Part print with two shaded views. Sizes in mm from the minimum x, y, z corner. A direction names the side the tool comes from. Round coordinates to 2 decimals unless told otherwise and drop trailing zeros. Loops run counter-clockwise (first coordinate to the right, second up) from the corner with the lowest first, then second, coordinate; pieces in that order, holes last. Notation, with made-up numbers: M -28,-9.75 L -18,-9.75 A38 cw -18,29.25 Z; hole C 65.25,23.5 d7. An arc over 180 degrees is marked long. Use a Markdown table: item, result. Add a question column.
Item 1: Saw through at D-D on z = 24.13. Write the cut outline in (x, y) (1 decimal).
Item 2: Saw through at C-C on z = 36.5. Write the cut outline in (x, y) (1 decimal).
Item 3: Saw through at A-A on z = 30.48. Write the cut outline in (x, y) (1 decimal).
Item 4: Pin check, flat tips, straight feed: P1, Ø8, axis at x = 36.5, z = 34.5, coming from the -Y side; P2, Ø3.5, axis at x = 52, y = 37.5, coming from the -Z side; P3, Ø12.5, axis at y = 11, z = 20, coming from the -X side; P4, Ø11.5, axis at x = 17.5, z = 34, coming from the -Y side. Stop position of each tip, or through.
Item 5: Wall check: L1, parallel to Y at x = 40, z = 24 (1 decimal); L2, parallel to Y at x = 52.35, z = 43.18 (1 decimal); L3, parallel to X at y = 34, z = 46 (1 decimal). Give the ranges that are in metal, low to high. Write a range as from..to.
Item 6: Tool access for the marked faces 1, 2, 3 and 4: list every direction of +Z, -Z, +X, -X, +Y, -Y with a clear straight run to the whole face (end or side of a thin tool).
Item 7: Saw through at B-B on y = 12.7. Write the cut outline in (x, z) (1 decimal).
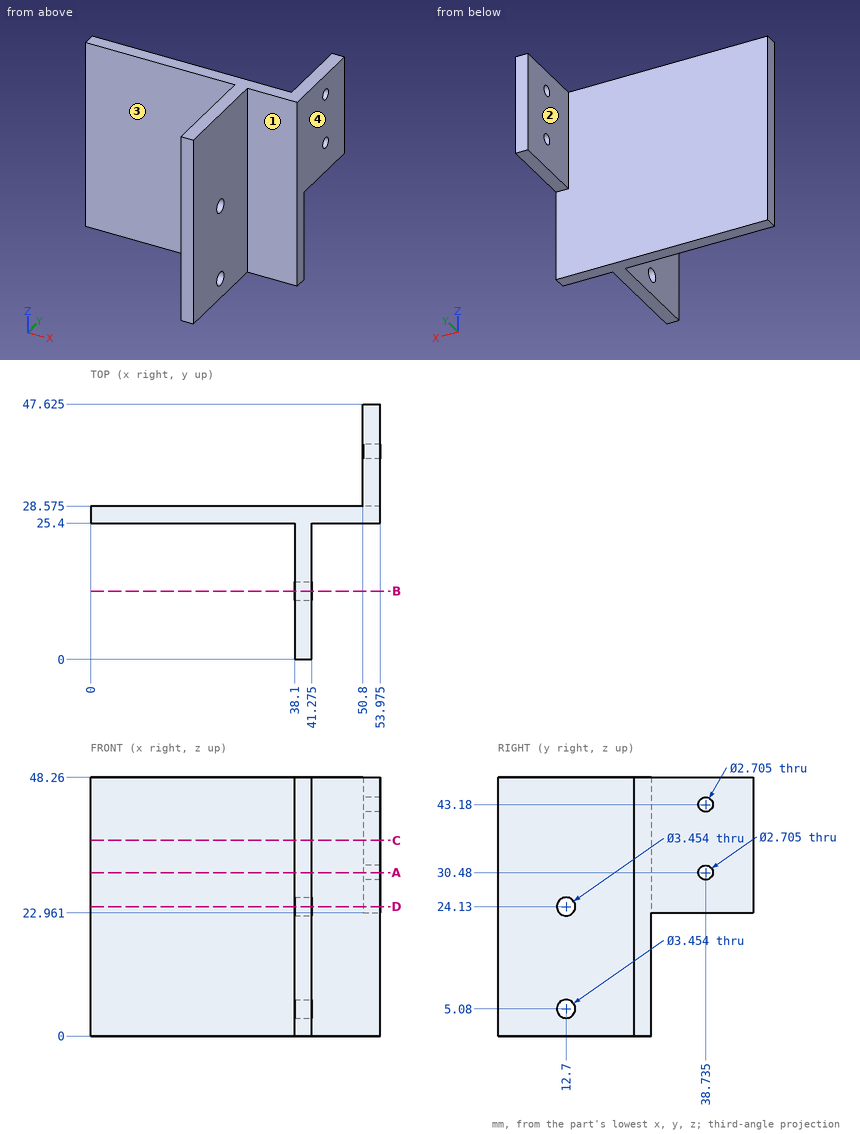
Entries:
| question | item | result |
|---|---|---|
| 1 | outline | M 0,25.4 L 38.1,25.4 L 38.1,14.4 L 41.3,14.4 L 41.3,25.4 L 54,25.4 L 54,47.6 L 50.8,47.6 L 50.8,28.6 L 0,28.6 Z; M 38.1,0 L 41.3,0 L 41.3,11 L 38.1,11 Z |
| 2 | outline | M 0,25.4 L 38.1,25.4 L 38.1,0 L 41.3,0 L 41.3,25.4 L 54,25.4 L 54,47.6 L 50.8,47.6 L 50.8,28.6 L 0,28.6 Z |
| 3 | outline | M 0,25.4 L 38.1,25.4 L 38.1,0 L 41.3,0 L 41.3,25.4 L 54,25.4 L 54,37.4 L 50.8,37.4 L 50.8,28.6 L 0,28.6 Z; M 50.8,40.1 L 54,40.1 L 54,47.6 L 50.8,47.6 Z |
| 4 | P1 | y = 0 |
| 4 | P2 | z = 22.96 |
| 4 | P3 | x = 38.1 |
| 4 | P4 | y = 25.4 |
| 5 | L1 | 0..11, 14.4..28.6 |
| 5 | L2 | 25.4..37.4, 40.1..47.6 |
| 5 | L3 | 50.8..54 |
| 6 | face 1 | +Z, -Z, +X, -Y |
| 6 | face 2 | +Z, -Z, -X, +Y |
| 6 | face 3 | +Z, -Z, -X, -Y |
| 6 | face 4 | +Z, -Z, +X, +Y, -Y |
| 7 | outline | M 38.1,0 L 41.3,0 L 41.3,3.4 L 38.1,3.4 Z; M 38.1,6.8 L 41.3,6.8 L 41.3,22.4 L 38.1,22.4 Z; M 38.1,25.9 L 41.3,25.9 L 41.3,48.3 L 38.1,48.3 Z |
